Autodesk Inventor part; units mm, degrees
ref_plane "YZ Plane" through (0, 0, 0) normal (1, 0, 0) x (0, 1, 0)
ref_plane "XZ Plane" through (0, 0, 0) normal (0, 1, 0) x (-1, 0, 0)
ref_plane "XY Plane" through (0, 0, 0) normal (0, 0, 1) x (1, 0, 0)
ref_plane "Work Plane1" through (0, 0, -4) normal (0, 0, 1) x (1, 0, 0)
sketch "Sketch1" plane through (0, 0, -4) normal (0, 0, 1) x (1, 0, 0)
  circle A0 centre (0.1176, -0.1618) radius 38.1
  circle A1 centre (0, 0) radius 43.6
  circle A2 centre (0, 0) radius 55.6
  point P0 (0, 0)
extrude "Extrusion1" add sketch "Sketch1" along normal blind 1 contours A1 | A2
sketch "Sketch2" plane through (0, 0, -3) normal (0, 0, 1) x (1, 0, 0)
  circle A0 centre (47.1724, 15.3272) radius 2
  circle A1 centre (47.1724, 15.3272) radius 4.4912
  line L0 (45.1335, 11.3256) -> (55.2569, 6.1675)
  circle A2 centre (0, 0) radius 55.6
  line L1 (43.1708, 17.3662) -> (48.3289, 27.4896)
  line L2 (47.1724, 15.3272) -> (52.8787, 17.1813)
  point P0 (0, 0)
  dimension "d2" = 45
  dimension "d3" = 45
extrude "Extrusion2" cut sketch "Sketch2" against normal blind 1 contours A0 | A1 | A1 L1 A2 L2 | L2 A2 L0 A1
fillet "Fillet1" radius 4 2 edges at (48.3289, 27.4896, -3.5) (55.2569, 6.1675, -3.5)
pattern_circular "Circular Pattern1" count 10 over 360 about axis through (0, 0, -4) along (0, 0, 1) of "Extrusion2", "Fillet1"
sketch "Sketch3" plane through (0, 0, -3) normal (0, 0, 1) x (1, 0, 0)
  arc A0 (47.1551, -29.4578) -> (47.3266, -25.5226) centre (43.7626, -27.3385) ccw
  line L0 (47.3266, -25.5226) -> (43.1708, -17.3662)
  arc A1 (45.1335, -11.3256) -> (43.1708, -17.3662) centre (47.1724, -15.3272) ccw
  line L1 (45.1335, -11.3256) -> (53.2898, -7.1697)
  arc A2 (53.2898, -7.1697) -> (55.4641, -3.8852) centre (51.4739, -3.6057) ccw
  arc A3 (55.4641, -3.8852) -> (55.4641, 3.8852) centre (0, 0) ccw
  arc A4 (55.4641, 3.8852) -> (53.2898, 7.1697) centre (51.4739, 3.6057) ccw
  line L2 (53.2898, 7.1697) -> (45.1335, 11.3256)
  arc A5 (43.1708, 17.3662) -> (45.1335, 11.3256) centre (47.1724, 15.3272) ccw
  line L3 (43.1708, 17.3662) -> (47.3266, 25.5226)
  arc A6 (47.3266, 25.5226) -> (47.1551, 29.4578) centre (43.7626, 27.3385) ccw
  arc A7 (47.1551, 29.4578) -> (42.5877, 35.7442) centre (0, 0) ccw
  arc A8 (42.5877, 35.7442) -> (38.8981, 37.1234) centre (39.5239, 33.1726) ccw
  line L4 (38.8981, 37.1234) -> (29.8567, 35.6914)
  arc A9 (24.7183, 39.4247) -> (29.8567, 35.6914) centre (29.1541, 40.1272) ccw
  line L5 (24.7183, 39.4247) -> (23.2863, 48.4661)
  arc A10 (23.2863, 48.4661) -> (20.8344, 51.5489) centre (19.3355, 47.8403) ccw
  arc A11 (20.8344, 51.5489) -> (13.4443, 53.9501) centre (0, 0) ccw
  arc A12 (13.4443, 53.9501) -> (9.6487, 52.8972) centre (12.4771, 50.0688) ccw
  line L6 (9.6487, 52.8972) -> (3.1757, 46.4243)
  arc A13 (-3.1757, 46.4243) -> (3.1757, 46.4243) centre (0, 49.6) ccw
  line L7 (-3.1757, 46.4243) -> (-9.6487, 52.8972)
  arc A14 (-9.6487, 52.8972) -> (-13.4443, 53.9501) centre (-12.4771, 50.0688) ccw
  arc A15 (-13.4443, 53.9501) -> (-20.8344, 51.5489) centre (0, 0) ccw
  arc A16 (-20.8344, 51.5489) -> (-23.2863, 48.4661) centre (-19.3355, 47.8403) ccw
  line L8 (-23.2863, 48.4661) -> (-24.7183, 39.4247)
  arc A17 (-29.8567, 35.6914) -> (-24.7183, 39.4247) centre (-29.1541, 40.1272) ccw
  line L9 (-29.8567, 35.6914) -> (-38.8981, 37.1234)
  arc A18 (-38.8981, 37.1234) -> (-42.5877, 35.7442) centre (-39.5239, 33.1726) ccw
  arc A19 (-42.5877, 35.7442) -> (-47.1551, 29.4578) centre (0, 0) ccw
  arc A20 (-47.1551, 29.4578) -> (-47.3266, 25.5226) centre (-43.7626, 27.3385) ccw
  line L10 (-47.3266, 25.5226) -> (-43.1708, 17.3662)
  arc A21 (-45.1335, 11.3256) -> (-43.1708, 17.3662) centre (-47.1724, 15.3272) ccw
  line L11 (-45.1335, 11.3256) -> (-53.2898, 7.1697)
  arc A22 (-53.2898, 7.1697) -> (-55.4641, 3.8852) centre (-51.4739, 3.6057) ccw
  arc A23 (-55.4641, 3.8852) -> (-55.4641, -3.8852) centre (0, 0) ccw
  arc A24 (-55.4641, -3.8852) -> (-53.2898, -7.1697) centre (-51.4739, -3.6057) ccw
  line L12 (-53.2898, -7.1697) -> (-45.1335, -11.3256)
  arc A25 (-43.1708, -17.3662) -> (-45.1335, -11.3256) centre (-47.1724, -15.3272) ccw
  line L13 (-43.1708, -17.3662) -> (-47.3266, -25.5226)
  arc A26 (-47.3266, -25.5226) -> (-47.1551, -29.4578) centre (-43.7626, -27.3385) ccw
  arc A27 (-47.1551, -29.4578) -> (-42.5877, -35.7442) centre (0, 0) ccw
  arc A28 (-42.5877, -35.7442) -> (-38.8981, -37.1234) centre (-39.5239, -33.1726) ccw
  line L14 (-38.8981, -37.1234) -> (-29.8567, -35.6914)
  arc A29 (-24.7183, -39.4247) -> (-29.8567, -35.6914) centre (-29.1541, -40.1272) ccw
  line L15 (-24.7183, -39.4247) -> (-23.2863, -48.4661)
  arc A30 (-23.2863, -48.4661) -> (-20.8344, -51.5489) centre (-19.3355, -47.8403) ccw
  arc A31 (-20.8344, -51.5489) -> (-13.4443, -53.9501) centre (0, 0) ccw
  arc A32 (-13.4443, -53.9501) -> (-9.6487, -52.8972) centre (-12.4771, -50.0688) ccw
  line L16 (-9.6487, -52.8972) -> (-3.1757, -46.4243)
  arc A33 (3.1757, -46.4243) -> (-3.1757, -46.4243) centre (0, -49.6) ccw
  line L17 (3.1757, -46.4243) -> (9.6487, -52.8972)
  arc A34 (9.6487, -52.8972) -> (13.4443, -53.9501) centre (12.4771, -50.0688) ccw
  arc A35 (13.4443, -53.9501) -> (20.8344, -51.5489) centre (0, 0) ccw
  arc A36 (20.8344, -51.5489) -> (23.2863, -48.4661) centre (19.3355, -47.8403) ccw
  line L18 (23.2863, -48.4661) -> (24.7183, -39.4247)
  arc A37 (29.8567, -35.6914) -> (24.7183, -39.4247) centre (29.1541, -40.1272) ccw
  line L19 (29.8567, -35.6914) -> (38.8981, -37.1234)
  arc A38 (38.8981, -37.1234) -> (42.5877, -35.7442) centre (39.5239, -33.1726) ccw
  arc A39 (42.5877, -35.7442) -> (47.1551, -29.4578) centre (0, 0) ccw
  circle A40 centre (0.1176, -0.1618) radius 38.1
  point P0 (0, 0)
equation "\"d3\" = d2"
properties part number "Anglerfish_3inch_tube_rubberring"
CAD build for the part. Positions are in the model's coordinates, mm. A direction names the side the tool comes from. Give positions to 0.01 mm unless a question says otherwise; leave off trailing zeros. Write each loop counter-clockwise with the first axis right and the second up, starting at its lowest first coordinate (ties: lowest second). Pieces come first, ordered by that corner, then holes. Notation, with made-up numbers: (37.5, -29.75) -> (73.5, -29.75) arc R28 ccw to (73.5, 8.25) -> close; hole circle Ø11 at (-14, 9). An arc over 180 degrees is marked (long way). Return JSON: item names as keys, results as strings.
Item 1: Drill centre lines: probe 1 along Y at (x, z) = (46, -3.05); probe 2 along X at (y, z) = (32.5, -3.75); probe 3 along X at (y, z) = (24, -3.05). Where is each one in solid material? Low to high.
Answer below:
{"probe 1": "y = -31.23 to -22.92, -10.88 to 10.88, 22.92 to 31.23", "probe 2": "x = -45.11 to -19.5, 19.73 to 45.11", "probe 3": "x = -46.55 to -29.34, 29.58 to 46.55"}
Item 2: Tool access for faces 1 (the cylindrical face through (17.233, -52.862, -3.507)), 2 (the flat face through (-49.15, -9.28, -3.49)), 3 (the flat face through (49.15, 9.28, -3.49)): list every direction of +Z, -Z, +X, -X, +Y, -Y with a clear straight run to the whole face (end or side of a thin tool).
Answer below:
{"face 1": "+Z, -Z, +X, -Y", "face 2": "+Z, -Z, -X", "face 3": "+Z, -Z, +X"}
Item 3: Two-plate mould, pull along X, no slides. Class faces 4 (the flat face through (-13, 36, -3)), 5 (the flat face through (-6.37, 49.62, -3.49)), 6 (the flat face through (45.22, 21.39, -3.49)): +X half, -X half, draft (parallel to the pull), parting line (faces both ways), or undercut.
Answer below:
{"face 4": "draft", "face 5": "undercut", "face 6": "+X half"}
Item 4: Band-saw the part on A-A (x = -6). List the corners of the cut face in (y, z).
Answer below:
{"outline": "(-49.25, -4) -> (-37.77, -4) -> (-37.77, -3) -> (-49.25, -3) -> close; (37.44, -4) -> (49.25, -4) -> (49.25, -3) -> (37.44, -3) -> close"}
